Geometry: see drawing. Coordinates: mm, zero at the bounding-box minimum. A direction names the side the tool comes from. Give positions to 0.01 mm unless a question says otherwise; leave off trailing zeros. Loops run counter-clockwise (first coordinate to the right, second up) from the corner with the lowest first, then second, coordinate; pieces in that order, holes last. Notation, with made-up numbers: M 81,37.5 L 133,37.5 A31 ccw 133,67.5 Z; hole C -35,-40 d6. An arc over 180 degrees is marked long. Return JSON: item names as keys, results as strings. Group by question number.
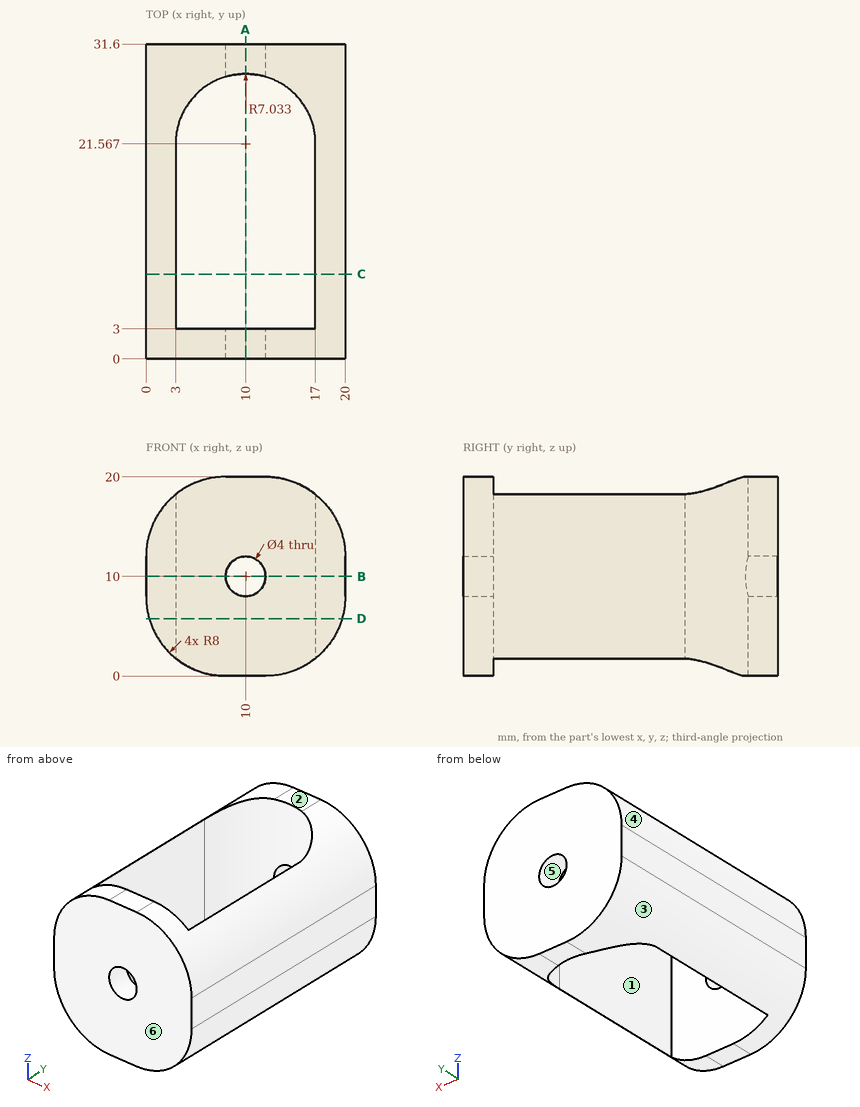
Item 1: Reachability of the marked faces 1 and 2 from +Z, -Z, +X, -X, +Y, -Y: full face, straight path, thin tool, end or side. Return the list, or none.
Item 2: Section B-B, the plane z = 10. Return loops of the section in (x, y).
Item 3: First-contact query: pin 1 Ø1 at (y, z) = (27.5, 6.5) entering from -X; pin 2 Ø3 at (x, y) = (16, 23.5) entering from -Z; pin 3 Ø5 at (x, y) = (5, 26) entering from +Z. Flat tips, straight axial feed; report the tip coordinate or a pass-through.
Item 4: Pull-direction query (Z, two-part tool) for the marked faces 3, 4, 5 and 6; classes: pulls with the +Z half, pulls with the -Z half, needs draft (parallel to the pull), parting line crosses it, or undercut.
Item 5: Material intervals for line 1 (X direction, y = 29.65, z = 10); line 2 (Y direction, x = 10.25, z = 5.5) (1 decimal); line 3 (X direction, y = 5.5, z = 9.5), sorted ascending. Write a range as from..to.
Item 6: Section A-A, the plane x = 10. Return loops of the section in (y, z).
Item 7: Section D-D, the plane z = 5.75. Return loops of the section in (x, y), then the cut area to 3 significant figures.
Item 8: Section C-C, the plane y = 8.5. Return loops of the section in (x, z) (1 decimal).
Answer below:
{
 "1": {"face 1": "+Z, -Z", "face 2": "+Z, +X, -X, +Y, -Y"},
 "2": {"outline": "M 0,0 L 8,0 L 8,3 L 3,3 L 3,22.25 A7.03 cw 8,28.31 L 8,31.6 L 0,31.6 Z; M 12,0 L 20,0 L 20,31.6 L 12,31.6 L 12,28.31 A7.03 cw 17,22.25 L 17,3 L 12,3 Z"},
 "3": {"pin 1": "x = 0.06", "pin 2": "z = 1.16", "pin 3": "z = 19.9"},
 "4": {"face 3": "pulls with the -Z half", "face 4": "pulls with the +Z half", "face 5": "undercut", "face 6": "needs draft"},
 "5": {"line 1": "0..8, 12..20", "line 2": "0..3, 28.6..31.6", "line 3": "0..3, 17..20"},
 "6": {"outline": "M 0,0 L 3,0 L 3,8 L 0,8 Z; M 0,12 L 3,12 L 3,20 L 0,20 Z; M 28.6,0 L 31.6,0 L 31.6,8 L 28.6,8 Z; M 28.6,12 L 31.6,12 L 31.6,20 L 28.6,20 Z"},
 "7": {"outline": "M 0.32,0 L 19.68,0 L 19.68,31.6 L 0.32,31.6 Z; hole M 3,3 L 17,3 L 17,22.25 A7.03 ccw 3,22.25 Z", "area": "274 mm^2"},
 "8": {"outline": "M 0,8 A8 ccw 3,1.8 L 3,18.2 A8 ccw 0,12 Z; M 17,1.8 A8 ccw 20,8 L 20,12 A8 ccw 17,18.2 Z"}
}
